For this review, take the finished solid that the model builds, in its own axes (mm). A direction names the side the tool comes from. Coordinates: 2 decimals unless noted, no trailing zeros. Order: outer loops, then holes, each group sorted by start corner. A loop starts at its lowest first (then second) coordinate and runs counter-clockwise, first axis right, second up. Notation, with made-up numbers: (33.25, -22) - (87.25, -22) arc R23 cw to (87.25, 5) - close; hole circle Ø4 at (28, -4). An arc over 180 degrees is marked (long way). One line per item, written item: value. Start each with the question number.
(1) Clearance check with flat-ended pins moving along their axes: pin 1 (4 mm diameter, centred on y = 17.5, z = -3, fed in from -X); pin 2 (4 mm diameter, centred on x = -3.5, y = 14.5, fed in from +Z); pin 3 (1.5 mm diameter, centred on x = -1.5, y = 31.5, fed in from +Z). State where each tip first meets the part, or that it passes through.
(2) For faces 1 (the conical face through (2.041, 0.086, 3.554)), 2 (the cylindrical face through (-2.44, 28.6, -0.54)), list the 3-axis set-ups (+Z, -Z, +X, -X, +Y, -Y) from which the entire face can be reached by the end or side of a thin tool; tool diameter is ignored.
(3) Consider section A-A on y = 48. Write out the cut boundary in (x, z), then the cut area to 3 significant figures.
(4) To check wall thickness, follow line 1 along Y through (x, z) = (1.5, 2.75); line 2 along Z through (x, y) = (1, 29). State the ranges of each line that lie inside material, in increasing order.
```python
from build123d import *

# Parameters (mm, degrees)
BOSS_EXTRUDE1_DEPTH = 53.5
SKETCH2_OUTSIDE_W   = 22.09
SKETCH2_OUTSIDE_H   = 20.868
SKETCH2_OUTSIDE_R   = 2.5
CUT_EXTRUDE1_DEPTH  = 50
CHAMFER1_SIZE       = 0.5


with BuildPart() as part:
    # Sketch1 → Boss-Extrude1 (new body)
    with BuildSketch(Plane(origin=(0, 0, 0), x_dir=(1, 0, 0), z_dir=(0, 1, 0))):
        Polygon((4.561067127, 0), (2.280533563, 3.95), (-2.280533563, 3.95), (-4.561067127, 0), (-2.280533563, -3.95), (2.280533563, -3.95), align=None)
    extrude(amount=BOSS_EXTRUDE1_DEPTH)

    # Sketch2 outside → Cut-Extrude1 (cut)
    with BuildSketch(Plane(origin=(0, 53.5, 0), x_dir=(1, 0, 0), z_dir=(0, 1, 0))):
        Rectangle(SKETCH2_OUTSIDE_W, SKETCH2_OUTSIDE_H)
        with Locations(Location((0, 0, 0), (0, 0, 270))):
            Circle(SKETCH2_OUTSIDE_R, mode=Mode.SUBTRACT)
    extrude(amount=-CUT_EXTRUDE1_DEPTH, mode=Mode.SUBTRACT)

    # Sketch3 → Cut-Revolve1 (revolve, cut)
    with BuildSketch(Plane(origin=(0, 0, 0), x_dir=(0, 0, -1), z_dir=(1, 0, 0))):
        Polygon((3.95, 0), (5.249038106, 0.75), (5.249038106, -0.75), align=None)
    revolve(axis=Axis((0, 3.5, 0), (0, 1, 0)), mode=Mode.SUBTRACT)

    # Chamfer1
    chamfer1_edges = [part.edges().sort_by_distance(p)[0] for p in [
        (0, 53.5, -2.5),
    ]]
    chamfer(chamfer1_edges, length=CHAMFER1_SIZE)


solid = part.part
```
Geometry check:
1. pin 1: stops at x = -2.29
1. pin 2: stops at z = 2
1. pin 3: stops at z = 2.38
2. face 1: +Z, +X, -Y
2. face 2: +Y
3. outline: circle Ø5 at (0, 0)
3. area: 19.6 mm^2
4. line 1: y = 0 to 3.5
4. line 2: z = -2.29 to 2.29
